Design review of the part built by this model. Coordinates are the model's own, in mm. A direction names the side the tool comes from. Round coordinates to 2 decimals unless told otherwise and drop trailing zeros. Write each loop counter-clockwise with the first axis right and the second up, starting at its lowest first coordinate (ties: lowest second). Pieces come first, ordered by that corner, then holes. Notation, with made-up numbers: M 83,-25.5 L 114,-25.5 A14 ccw 114,-18.5 Z; hole C 75.25,58 d11. An arc over 180 degrees is marked long. Use CSV: the item, a comma, the result in double quotes.
from build123d import *

# Parameters (mm, degrees)
SKETCH1_R           = 12.5
BOSS_EXTRUDE1_DEPTH = 66.71
SKETCH2_W           = 16.007
SKETCH2_H           = 19.203540064
BOSS_EXTRUDE2_DEPTH = 20
BOSS_EXTRUDE3_DEPTH = 16.007
SKETCH4_R           = 3
CUT_EXTRUDE1_DEPTH  = 71.900406291
SKETCH5_R           = 3
CUT_EXTRUDE2_DEPTH  = 15


with BuildPart() as part:
    # Sketch1 → Boss-Extrude1 (new body)
    with BuildSketch(Plane(origin=(0, 0, 0), x_dir=(0, 0, -1), z_dir=(1, 0, 0))):
        Circle(SKETCH1_R)
    extrude(amount=BOSS_EXTRUDE1_DEPTH)

    # Sketch2 → Boss-Extrude2 (add)
    with BuildSketch(Plane.ZY):
        Rectangle(SKETCH2_W, SKETCH2_H)
    extrude(amount=BOSS_EXTRUDE2_DEPTH)

    # Sketch3 → Boss-Extrude3 (add)
    with BuildSketch(Plane.XY.offset(8.0035)):
        with BuildLine():
            Line((-20, 9.601770032), (-20, -9.601770032))
            ThreePointArc((-20, -9.601770032), (-29.601770032, 0), (-20, 9.601770032))
        make_face()
    extrude(amount=-BOSS_EXTRUDE3_DEPTH)

    # Sketch4 → Cut-Extrude1 (cut, through all)
    with BuildSketch(Plane.XY.offset(8.0035)):
        with Locations((-20, 0)):
            Circle(SKETCH4_R)
    extrude(amount=-CUT_EXTRUDE1_DEPTH, mode=Mode.SUBTRACT)

    # Sketch5 → Cut-Extrude2 (cut)
    with BuildSketch(Plane(origin=(66.71, 0, 0), x_dir=(0, 0, -1), z_dir=(1, 0, 0))):
        Circle(SKETCH5_R)
    extrude(amount=-CUT_EXTRUDE2_DEPTH, mode=Mode.SUBTRACT)


solid = part.part
1) Add section D-D on x = -3.5. Write out the cut boundary in (y, z).
Answers:
outline,"M -9.6,-8 L 9.6,-8 L 9.6,8 L -9.6,8 Z"
2) Add section B-B on x = 25. Write out the cut boundary in (y, z), then the cut area to 3 significant figures.
Answers:
outline,"C 0,0 d25"
area,"491 mm²"
3) For pin 1 Ø5 at (y, z) = (-4, -11) entering from -X; pin 2 Ø8 at (x, z) = (-5, -3) entering from -Y; pin 3 Ø4 at (y, z) = (0, -9) entering from -X; pin 4 Ø3 at (x, y) = (35.5, 8) entering from -Z, all flat-tipped, find the tip position at first contact; note any pin that passes through.
Answers:
pin 1,"x = 0"
pin 2,"y = -9.6"
pin 3,"x = -29.6"
pin 4,"z = -10.68"
4) Add section A-A on z = 0. Write out the cut boundary in (x, y).
Answers:
outline,"M -20,-9.6 L 0,-9.6 L 0,-12.5 L 66.71,-12.5 L 66.71,-3 L 51.71,-3 L 51.71,3 L 66.71,3 L 66.71,12.5 L 0,12.5 L 0,9.6 L -20,9.6 A9.6 ccw Z; hole C -20,0 d6"
5) Wall thickness on line 1 along Y through (x, z) = (-20, -3.5); line 2 along Y through (x, z) = (57.5, 0); line 3 along Z through (x, y) = (54, 0.25): over which ranges is each line inside the solid? List them lowest first. Write a range as [from, to].
Answers:
line 1,"[-9.6, -3], [3, 9.6]"
line 2,"[-12.5, -3], [3, 12.5]"
line 3,"[-12.5, -2.99], [2.99, 12.5]"
6) The part is to be moulded in two halves that separate along Z. For faces 1 (the face through (-15, 0, 8.004)), 2 (the face through (-23, 0, 0)), 3 (the face through (59, 0, 3)), say which applies: released by +Z, released by -Z, zero draft, split by the parting line, or undercut.
Answers:
face 1,"released by +Z"
face 2,"zero draft"
face 3,"undercut"
7) Add section C-C on z = -10.25. Write out the cut boundary in (x, y).
Answers:
outline,"M 0,-7.15 L 66.71,-7.15 L 66.71,7.15 L 0,7.15 Z"
8) Machinability: for faces 4 (the face through (0, 0, 10)), 5 (the face through (-15, 0, -8.004)), 6 (the face through (51.71, 0, 0)), 7 (the face through (0, 11, 0)), 8 (the face through (0, -11, 0)), which of the approach directions +Z, -Z, +X, -X, +Y, -Y give a long, thin tool a straight path to every point of the face, cutting with its end or side? Answer none if there is none.
Answers:
face 4,"+Z, -X, +Y, -Y"
face 5,"-Z, -X, +Y, -Y"
face 6,"+X"
face 7,"+Z, -Z, -X, +Y"
face 8,"+Z, -Z, -X, -Y"
